from build123d import *

# Parameters (mm, degrees)
BOSS_EXTRUDE1_DEPTH = 3
SKETCH2_R           = 4.05
SKETCH2_R_2         = 2.55
CUT_EXTRUDE1_DEPTH  = 3
FILLET1_R           = 0.1


with BuildPart() as part:
    # Sketch1 → Boss-Extrude1 (new body)
    with BuildSketch(Plane(origin=(0, 0, 0), x_dir=(1, 0, 0), z_dir=(0, 1, 0))):
        with BuildLine():
            Line((50, -15), (-50, -15))
            ThreePointArc((-50, -15), (-65, 0), (-50, 15))
            Line((-50, 15), (-5.606634193, 15))
            Line((-5.606634193, 15), (-5.606634193, 50))
            Line((-5.606634193, 50), (0, 63.840242005))
            Line((0, 63.840242005), (5.606634193, 50))
            Line((5.606634193, 50), (5.606634193, 15))
            Line((5.606634193, 15), (50, 15))
            ThreePointArc((50, 15), (65, 0), (50, -15))
        make_face()
    extrude(amount=BOSS_EXTRUDE1_DEPTH)

    # Sketch2 → Cut-Extrude1 (cut)
    with BuildSketch(Plane(origin=(0, 3, 0), x_dir=(1, 0, 0), z_dir=(0, 1, 0))):
        with Locations(Location((0, 0, 0), (0, 0, 270))):
            Circle(SKETCH2_R)
        with Locations(Location((-50, 0, 0), (0, 0, 270))):
            Circle(SKETCH2_R_2)
        with Locations(Location((50, 0, 0), (0, 0, 90))):
            Circle(SKETCH2_R_2)
    extrude(amount=-CUT_EXTRUDE1_DEPTH, mode=Mode.SUBTRACT)

    # Fillet1
    fillet1_edges = [part.edges().sort_by_distance(p)[0] for p in [
        (0, 1.5, -63.840242005),
    ]]
    fillet(fillet1_edges, radius=FILLET1_R)


solid = part.part
CAD build for the part. Positions are in the model's coordinates, mm. A direction names the side the tool comes from. Give positions to 0.01 mm unless a question says otherwise; leave off trailing zeros. Write each loop counter-clockwise with the first axis right and the second up, starting at its lowest first coordinate (ties: lowest second). Pieces come first, ordered by that corner, then holes. Notation, with made-up numbers: (-28, 27.5) -> (9, 27.5) arc R30 ccw to (9, 59.5) -> close; hole circle Ø6 at (-17, 60). An arc over 180 degrees is marked (long way). Return JSON: item names as keys, results as strings.
Item 1: Drop flat-ended pins along their axis: pin 1 (0.9 mm diameter, centred on x = -26, y = 1, fed in from -Z); pin 2 (0.9 mm diameter, centred on y = 1.5, z = -30.5, fed in from +X). Give the stop position or say it passes through.
Answer below:
{"pin 1": "stops at z = -15", "pin 2": "stops at x = 5.61"}
Item 2: Band-saw the part on B-B (y = 0.85). List the corners of the cut face in (x, z).
Answer below:
{"outline": "(-50, -15) -> (-5.61, -15) -> (-5.61, -50) -> (-0.09, -63.61) arc R0.1 ccw to (0.09, -63.61) -> (5.61, -50) -> (5.61, -15) -> (50, -15) arc R15 ccw to (50, 15) -> (-50, 15) arc R15 ccw to start; hole circle Ø5.1 at (-50, 0); hole circle Ø8.1 at (0, 0); hole circle Ø5.1 at (50, 0)"}
Item 3: Drill centre lines: probe 1 along X at (y, z) = (2.25, 0); probe 2 along Z at (x, y) = (50, 0.85); probe 3 along X at (y, z) = (0.25, -47.5). Where is each one in solid material? Low to high.
Answer below:
{"probe 1": "x = -65 to -52.55, -47.45 to -4.05, 4.05 to 47.45, 52.55 to 65", "probe 2": "z = -15 to -2.55, 2.55 to 15", "probe 3": "x = -5.61 to 5.61"}
Item 4: Band-saw the part on A-A (z = 0). List the corners of the cut face in (x, y).
Answer below:
{"outline": "(-65, 0) -> (-52.55, 0) -> (-52.55, 3) -> (-65, 3) -> close; (-47.45, 0) -> (-4.05, 0) -> (-4.05, 3) -> (-47.45, 3) -> close; (4.05, 0) -> (47.45, 0) -> (47.45, 3) -> (4.05, 3) -> close; (52.55, 0) -> (65, 0) -> (65, 3) -> (52.55, 3) -> close"}
Item 5: Band-saw the part on D-D (x = 33). List the corners of the cut face in (y, z), then the cut area to 3 significant figures.
Answer below:
{"outline": "(0, -15) -> (3, -15) -> (3, 15) -> (0, 15) -> close", "area": "90.0 mm2"}
Item 6: Band-saw the part on C-C (z = -28). List the corners of the cut face in (x, y).
Answer below:
{"outline": "(-5.61, 0) -> (5.61, 0) -> (5.61, 3) -> (-5.61, 3) -> close"}
Item 7: Tool access for faces 4 (the flat face through (5.607, 1, -33)), 5 (the flat face through (-5.607, 1, -32)), 6 (the cylindrical face through (65, 1, 0)): list every direction of +Z, -Z, +X, -X, +Y, -Y with a clear straight run to the whole face (end or side of a thin tool).
Answer below:
{"face 4": "-Z, +X, +Y, -Y", "face 5": "-Z, -X, +Y, -Y", "face 6": "+X, +Y, -Y"}
Item 8: Two-plate mould, pull along Z, no slides. Class faces 1 (the flat face through (1, 0, -7)), 2 (the cylindrical face through (47.47, 1.52, 0.33)), 3 (the flat face through (2.81, 1.48, -56.9)): +Z half, -Z half, draft (parallel to the pull), parting line (faces both ways), or undercut.
Answer below:
{"face 1": "draft", "face 2": "undercut", "face 3": "-Z half"}
